Source: CAD feature listing. Evaluate the final solid. Frame: model axes, mm. Coordinates: 2 decimals unless noted, no trailing zeros. Order: outer loops, then holes, each group sorted by start corner. A loop starts at its lowest first (then second) coordinate and runs counter-clockwise, first axis right, second up. Notation, with made-up numbers: (29.25, 21) -> (61.25, 21) arc R35 ccw to (61.25, 56) -> close; hole circle Ø4 at (75.5, 6). An arc over 180 degrees is marked (long way). Put each result on its own line as item: value.
from build123d import *

# Parameters (mm, degrees)
F0_R     = 350
F0_R_2   = 20
F0_R_3   = 35
F1_DEPTH = 20


with BuildPart() as f1:
    # F0 (on Top) → F1 (new body)
    with BuildSketch(Plane.XY):
        Circle(F0_R)
        with Locations((-168.410354, -200.703644)):
            Circle(F0_R_2, mode=Mode.SUBTRACT)
        with Locations((-59.853525, -164.446209)):
            Circle(F0_R_2, mode=Mode.SUBTRACT)
        with Locations((-172.341357, -30.388431)):
            Circle(F0_R_2, mode=Mode.SUBTRACT)
        with Locations((-76.210236, -44)):
            Circle(F0_R_2, mode=Mode.SUBTRACT)
        with Locations((89.609278, -246.199467)):
            Circle(F0_R_2, mode=Mode.SUBTRACT)
        with Locations((0, -88)):
            Circle(F0_R_2, mode=Mode.SUBTRACT)
        with Locations((112.487832, -134.057778)):
            Circle(F0_R_2, mode=Mode.SUBTRACT)
        with Locations((76.210236, -44)):
            Circle(F0_R_2, mode=Mode.SUBTRACT)
        with Locations((258.019631, -45.495823)):
            Circle(F0_R_2, mode=Mode.SUBTRACT)
        with Locations((-258.019631, 45.495823)):
            Circle(F0_R_2, mode=Mode.SUBTRACT)
        with Locations((-76.210236, 44)):
            Circle(F0_R_2, mode=Mode.SUBTRACT)
        with Locations((-112.487832, 134.057778)):
            Circle(F0_R_2, mode=Mode.SUBTRACT)
        with Locations((-89.609278, 246.199467)):
            Circle(F0_R_2, mode=Mode.SUBTRACT)
        Circle(F0_R_3, mode=Mode.SUBTRACT)
        with Locations((76.210236, 44)):
            Circle(F0_R_2, mode=Mode.SUBTRACT)
        with Locations((172.341357, 30.388431)):
            Circle(F0_R_2, mode=Mode.SUBTRACT)
        with Locations((0, 88)):
            Circle(F0_R_2, mode=Mode.SUBTRACT)
        with Locations((59.853525, 164.446209)):
            Circle(F0_R_2, mode=Mode.SUBTRACT)
        with Locations((168.410354, 200.703644)):
            Circle(F0_R_2, mode=Mode.SUBTRACT)
    extrude(amount=F1_DEPTH)


solid = f1.part
1. Ray query, line 1 along Y through (x, z) = (0, 6); line 2 along X through (y, z) = (-0.5, 14.5); line 3 along Y through (x, z) = (-166, 15.75). Return the intervals inside material, ascending.
Numbers:
line 1: y = -350 to -108, -68 to -35, 35 to 68, 108 to 350
line 2: x = -350 to -35, 35 to 350
line 3: y = -308.13 to -220.56, -180.85 to -49.36, -11.42 to 308.13
2. First-contact query: pin 1 (3 mm diameter, centred on x = -216.5, z = 16.5, fed in from +Y); pin 2 (6 mm diameter, centred on y = -54, z = 12.5, fed in from -X); pin 3 (2 mm diameter, centred on x = -114.5, z = 11.5, fed in from -Y). Flat tips, straight axial feed; report the tip coordinate or a pass-through.
Numbers:
pin 1: stops at y = 276.18
pin 2: stops at x = -346.26
pin 3: stops at y = -331.09
3. Pull-direction query (Y, two-part tool) for faces 1 (the flat face through (73, 5, 20)), 2 (the cylindrical face through (78.93, 170.45, 9.86)), 3 (the cylindrical face through (-128.36, 121.89, 9.86)); classes: pulls with the +Y half, pulls with the -Y half, needs draft (parallel to the pull), parting line crosses it, or undercut.
Numbers:
face 1: needs draft
face 2: undercut
face 3: undercut
4. Cut plane D-D on z = 5.25. Count the separate pieces of the cut face and the enclosed holes in it, plus the area to 3 significant figures.
Numbers:
separate pieces: 1
enclosed holes: 19
area: 358,000 mm2
5. Cut plane A-A on y = 0. Output: boundary loops of the cut face in (x, z).
Numbers:
outline: (-350, 0) -> (-35, 0) -> (-35, 20) -> (-350, 20) -> close; (35, 0) -> (350, 0) -> (350, 20) -> (35, 20) -> close
6. Cut plane B-B on x = 0. Output: boundary loops of the cut face in (y, z), plus the area to 3 significant figures.
Numbers:
outline: (-350, 0) -> (-108, 0) -> (-108, 20) -> (-350, 20) -> close; (-68, 0) -> (-35, 0) -> (-35, 20) -> (-68, 20) -> close; (35, 0) -> (68, 0) -> (68, 20) -> (35, 20) -> close; (108, 0) -> (350, 0) -> (350, 20) -> (108, 20) -> close
area: 11,000 mm2
7. Cut plane C-C on x = 263.5. Output: boundary loops of the cut face in (y, z).
Numbers:
outline: (-230.36, 0) -> (-64.73, 0) -> (-64.73, 20) -> (-230.36, 20) -> close; (-26.26, 0) -> (230.36, 0) -> (230.36, 20) -> (-26.26, 20) -> close
